```python
from build123d import *

# Parameters (mm, degrees)
F0_R            = 101.6
F0_R_2          = 14.1605
F1_DEPTH        = 3.175
F2_R            = 2.3622
F3_DEPTH        = 3.176
F3_COPIES_COUNT = 6


# Not quite as in the source:
# - a pattern or mirror of a feature is missing from the dataset's text; its kind, count and spacing are read off the source's solid


with BuildPart() as f1:
    # F0 (on Top) → F1 (new body)
    with BuildSketch(Plane.XY):
        Circle(F0_R)
        Circle(F0_R_2, mode=Mode.SUBTRACT)
    extrude(amount=F1_DEPTH)

    # F2 (on face) → F3 (cut, through all)
    with BuildSketch(Plane.XY.offset(3.175)):
        with Locations((0, 23.8125)):
            Circle(F2_R)
        with Locations((0, 76.2)):
            Circle(F2_R)
        with Locations((25.4, 43.9940905122)):
            Circle(F2_R)
    f3 = extrude(amount=-F3_DEPTH, mode=Mode.SUBTRACT)

    # F3_copies: F3 ×6 about axis
    f3_copies_axis = Axis((0, 0, 0), (0, 0, 1))
    for i in range(1, F3_COPIES_COUNT):
        add(f3.rotate(f3_copies_axis, i * 360 / F3_COPIES_COUNT), mode=Mode.SUBTRACT)


solid = f1.part
```
Geometry: final body of the model. Coordinates: model frame, mm. Round coordinates to 2 decimals unless told otherwise and drop trailing zeros. Order: outer loops, then holes, each group sorted by start corner. A loop starts at its lowest first (then second) coordinate and runs counter-clockwise, first axis right, second up. Notation, with made-up numbers: M -10.5,2.5 L 46.5,2.5 A13 ccw 46.5,22.5 Z; hole C 14,61.5 d9. An arc over 180 degrees is marked long. Use one line per item in the form item = value. Start each with the question number.
Q1. Cut plane C-C (x = 77). Return loops of the section in (y, z) (3 decimals).
Q2. Material intervals for line 1 (Y direction, x = 0, z = 2.3); line 2 (Y direction, x = 22, z = 2.4); line 3 (Y direction, x = -25.4, z = 2), sorted ascending. Write a range as [from, to].
Q3. Cut plane D-D (y = 58). Return loops of the section in (x, z) (3 decimals).
Q4. Cut plane B-B (z = 2.55). Count the separate pieces of the cut face and the enclosed holes in it, and give its area (3 significant figures).
Q5. Cut plane A-A (x = 0). Return loops of the section in (y, z) (1 decimal), and give its area (3 significant figures).
Q6. Pin query (flat end, axial travel): pin 1 Ø1 at (y, z) = (62, 1) entering from +X. Return the tip coordinate at first contact, or that it passes through.
Q7. Mould query, pull axis Y, two halves, no side actions, for faces 1 (the face through (-22.025, -99.184, 1.565)), 2 (the face through (22.875, -11.197, 1.61)), 3 (the face through (21, 1, 0)), 4 (the face through (-22.875, 11.197, 1.61)). Classes: +Y half, -Y half, draft (parallel to the pull), parting line (faces both ways), or undercut.
Geometry results:
q1.outline = M -66.284,0 L 66.284,0 L 66.284,3.175 L -66.284,3.175 Z
q2.line_1 = [-101.6, -78.56], [-73.84, -26.17], [-21.45, -14.16], [14.16, 21.45], [26.17, 73.84], [78.56, 101.6]
q2.line_2 = [-99.19, -13.83], [-9.99, 9.99], [13.83, 99.19]
q2.line_3 = [-98.37, -46.36], [-41.63, 41.63], [46.36, 98.37]
q3.outline = M -83.418,0 L 83.418,0 L 83.418,3.175 L -83.418,3.175 Z
q4.separate_pieces = 1
q4.enclosed_holes = 19
q4.area = 31,500 mm^2
q5.outline = M -101.6,0 L -78.6,0 L -78.6,3.2 L -101.6,3.2 Z; M -73.8,0 L -26.2,0 L -26.2,3.2 L -73.8,3.2 Z; M -21.5,0 L -14.2,0 L -14.2,3.2 L -21.5,3.2 Z; M 14.2,0 L 21.5,0 L 21.5,3.2 L 14.2,3.2 Z; M 26.2,0 L 73.8,0 L 73.8,3.2 L 26.2,3.2 Z; M 78.6,0 L 101.6,0 L 101.6,3.2 L 78.6,3.2 Z
q5.area = 495 mm^2
q6.pin_1 = 80.87
q7.face_1 = parting line
q7.face_2 = undercut
q7.face_3 = draft
q7.face_4 = undercut
